Autodesk Inventor part; units mm, degrees
ref_plane "YZ Plane" through (0, 0, 0) normal (1, 0, 0) x (0, 1, 0)
ref_plane "XZ Plane" through (0, 0, 0) normal (0, 1, 0) x (-1, 0, 0)
ref_plane "XY Plane" through (0, 0, 0) normal (0, 0, 1) x (1, 0, 0)
sketch "Skizze2" plane through (0, 0, 0) normal (1, 0, 0) x (0, 1, 0)
  line L0 (13, 0) -> (0, 0)
  line L1 (3, 4) -> (0, 4)
  line L2 (0, 4) -> (0, 0)
  line L3 (5.9544, 6.4791) -> (13.1736, 5.2061)
  line L4 (13.1736, 5.2061) -> (5.9544, 6.4791)
  arc A0 (3, 4) -> (5.9544, 6.4791) centre (3, 7) ccw
  arc A1 (13.5, 3.3553) -> (13.1736, 5.2061) centre (13, 4.2213) ccw
  arc A2 (13.5, 3.3553) -> (13, 2.4893) centre (14, 2.4893) ccw
  line L5 (13, 2.4893) -> (13, 0)
  dimension "d3" = 80
  dimension "d4" = 4
  dimension "d5" = 13
  dimension "d7" = 3
  dimension "d8" = 1
  dimension "d9" = 3
  dimension "d10" = 0
revolve "Umdrehung1" add sketch "Skizze2" angle 360 about axis through (0, 13, 0) along (0, -1, 0)
sketch "Skizze1" plane through (0, 0, 0) normal (0, 1, 0) x (-1, 0, 0)
  arc A0 (-1.1779, 0.55) -> (1.1779, 0.55) centre (0, 0) ccw
  line L0 (-1.1779, 0.55) -> (1.1779, 0.55)
  dimension "d0" = 1.3
  dimension "d1" = 0.55
extrude "Extrusion1" cut sketch "Skizze1" along normal blind 6
sketch "Skizze3" plane through (0, 0, 0) normal (0, -1, 0) x (1, 0, 0)
  arc A0 (-1.1779, 0.55) -> (1.1779, 0.55) centre (0, 0) ccw
  circle A1 centre (0, 0) radius 1.5
  point P0 (0, 0)
  dimension "d14" = 3
extrude "Extrusion2" cut sketch "Skizze3" against normal blind 1
fillet "Rundung1" radius 2 1 edges at (0, 5.9544, -6.4791)
properties part number "_3D-Druck"
CAD build for the part. Positions are in the model's coordinates, mm. A direction names the side the tool comes from. Give positions to 0.01 mm unless a question says otherwise; leave off trailing zeros. Loops run counter-clockwise (first coordinate to the right, second up) from the corner with the lowest first, then second, coordinate; pieces in that order, holes last. Notation, with made-up numbers: M 41.25,41 L 64.25,41 A17 cw 64.25,54 Z; hole C 18,-18.5 d9. An arc over 180 degrees is marked long. One line per question, with ' | ' between items. Start each with the question number.
1. Saw through at A-A on y = 2. Give the cut face in (x, z).
2. Flat gauge pins, fed straight in: pin 1 (6 mm diameter, centred on y = 4, z = -1, fed in from -X); pin 2 (1.9 mm diameter, centred on x = -0.5, y = 2.5, fed in from -Z); pin 3 (2 mm diameter, centred on x = 0, z = 0, fed in from -Y). Where does each tip first touch, or does it go through?
3. Probe L1, parallel to X at y = 2.55, z = 0; L2, parallel to Y at x = -1.75, z = -2.5; L3, parallel to Y at x = 1.75, z = -1.5. List the from-to ranges inside material, lowest first. Write a range as from..to.
4. Two-plate mould, pull along Z, no slides. Class faces 3 (the face through (3.905, 1.479, -0.867)), 4 (the face through (-1.5, 0.49, 0.07)), 5 (the face through (0, 0, 2)): pulls with the +Z half, pulls with the -Z half, needs draft (parallel to the pull), parting line crosses it, or undercut.
5. 3-axis set-ups, long thin cutter, end or side, ignore diameter. For faces 1 (the face through (0, 3, 0.55)), 2 (the face through (0, 13, 0)): which of +Z, -Z, +X, -X, +Y, -Y reach the whole face in a straight line?
Result sheet:
1) outline: C 0,0 d8; hole M -1.18,0.55 A1.3 ccw long 1.18,0.55 Z
2) pin 1: stops at x = -6.21 | pin 2: stops at z = -4.02 | pin 3: stops at y = 1
3) L1: x = -4..-1.3, 1.3..4 | L2: y = 0..13.17 | L3: y = 0..13
4) face 3: parting line crosses it | face 4: undercut | face 5: needs draft
5) face 1: -Y | face 2: +Y
